Here's how the part is built. I have some questions about the finished solid (model axes, mm). Face numbers are marked on the shaded views. A direction names the side the tool comes from. Coordinates: 2 decimals unless noted, no trailing zeros. Loops run counter-clockwise (first coordinate to the right, second up) from the corner with the lowest first, then second, coordinate; pieces in that order, holes last. Notation, with made-up numbers: (51, -7.5) -> (62, -7.5) arc R7 ccw to (62, 0.5) -> close; hole circle Ø10 at (1.5, -30). An arc over 180 degrees is marked (long way). Answer as a JSON object with one key per item and string values. Group by question number.
Q1. I'm going to push flat-ended pins straight in: pin 1 (2 mm diameter, centred on y = 3, z = 4, fed in from +X); pin 2 (3.5 mm diameter, centred on x = -1, y = -1, fed in from +Z); pin 3 (3 mm diameter, centred on y = -2.5, z = 2.5, fed in from -X); pin 4 (1.8 mm diameter, centred on x = 17, y = 0, fed in from -Z). Where does each tip first touch, or does it pass through?
Q2. I want a section at D-D on z = 2.75. Write out the boundary of the cut face in (x, y), then the cut area to 3 significant figures.
Q3. I want a section at B-B on y = 0. Write out the boundary of the cut face in (x, z).
Q4. On a 3-axis mill with a long thin cutter (end or side, diameter ignored), from which of +Z, -Z, +X, -X, +Y, -Y can I reach the whole of each face in a straight line? I mean the marked faces 4 and 5. Say none if no direction works.
Q5. I want a section at C-C on x = 17. Write out the boundary of the cut face in (y, z).
Q6. Thinking about a two-plate mould opening in X: for the marked faces 1, 2 and 3, which applies, released by +X, released by -X, zero draft, split by the parting line, or undercut?
Q7. I need wall thicknesses on line 1 (Y direction, x = 0, z = 1.4); line 2 (Y direction, x = 0, z = 4.1); line 3 (X direction, y = -1.75, z = 2.65). Which ranges of each line are inside material? Lowest first, please.
Q8. I want a section at A-A on z = 1.05. Write out the boundary of the cut face in (x, y).
```python
from build123d import *

# Parameters (mm, degrees)
SKETCH1_R           = 1.5
BOSS_EXTRUDE1_DEPTH = 2
SKETCH2_R           = 4.5
SKETCH2_R_2         = 3.5
BOSS_EXTRUDE2_DEPTH = 3
SKETCH3_R           = 1
CUT_EXTRUDE1_DEPTH  = 3


with BuildPart() as part:
    # Sketch1 → Boss-Extrude1 (new body)
    with BuildSketch(Plane.XY):
        with BuildLine():
            Line((-17.442345164, 2.460554969), (-3.31662479, 5))
            ThreePointArc((-3.31662479, 5), (0, 6), (3.31662479, 5))
            Line((3.31662479, 5), (17.442345164, 2.460554969))
            ThreePointArc((17.442345164, 2.460554969), (19.5, 0), (17.442345164, -2.460554969))
            Line((17.442345164, -2.460554969), (3.31662479, -5))
            ThreePointArc((3.31662479, -5), (0, -6), (-3.31662479, -5))
            Line((-3.31662479, -5), (-17.442345164, -2.460554969))
            ThreePointArc((-17.442345164, -2.460554969), (-19.5, 0), (-17.442345164, 2.460554969))
        make_face()
        Circle(SKETCH1_R, mode=Mode.SUBTRACT)
    extrude(amount=BOSS_EXTRUDE1_DEPTH)

    # Sketch2 → Boss-Extrude2 (add)
    with BuildSketch(Plane.XY.offset(2)):
        Circle(SKETCH2_R)
        Circle(SKETCH2_R_2, mode=Mode.SUBTRACT)
    extrude(amount=BOSS_EXTRUDE2_DEPTH)

    # Sketch3 → Cut-Extrude1 (cut, through all)
    with BuildSketch(Plane.XY.offset(2)):
        with Locations((-17, 0)):
            Circle(SKETCH3_R)
        with Locations((17, 0)):
            Circle(SKETCH3_R)
    extrude(amount=-CUT_EXTRUDE1_DEPTH, mode=Mode.SUBTRACT)


solid = part.part
```
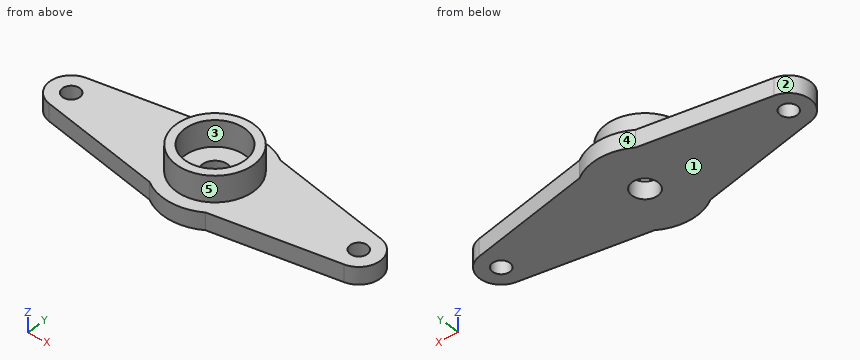
Result set:
{
 "1": {"pin 1": "stops at x = 4.03", "pin 2": "stops at z = 2", "pin 3": "stops at x = -19.25", "pin 4": "passes through"},
 "2": {"outline": "circle Ø9 at (0, 0); hole circle Ø7 at (0, 0)", "area": "25.1 mm²"},
 "3": {"outline": "(-19.5, 0) -> (-18, 0) -> (-18, 2) -> (-19.5, 2) -> close; (-16, 0) -> (-1.5, 0) -> (-1.5, 2) -> (-3.5, 2) -> (-3.5, 5) -> (-4.5, 5) -> (-4.5, 2) -> (-16, 2) -> close; (1.5, 0) -> (16, 0) -> (16, 2) -> (4.5, 2) -> (4.5, 5) -> (3.5, 5) -> (3.5, 2) -> (1.5, 2) -> close; (18, 0) -> (19.5, 0) -> (19.5, 2) -> (18, 2) -> close"},
 "4": {"face 4": "+Z, -Z, +Y", "face 5": "+Z"},
 "5": {"outline": "(-2.54, 0) -> (-1, 0) -> (-1, 2) -> (-2.54, 2) -> close; (1, 0) -> (2.54, 0) -> (2.54, 2) -> (1, 2) -> close"},
 "6": {"face 1": "zero draft", "face 2": "released by -X", "face 3": "undercut"},
 "7": {"line 1": "y = -6 to -1.5, 1.5 to 6", "line 2": "y = -4.5 to -3.5, 3.5 to 4.5", "line 3": "x = -4.15 to -3.03, 3.03 to 4.15"},
 "8": {"outline": "(-17.44, -2.46) -> (-3.32, -5) arc R6 ccw to (3.32, -5) -> (17.44, -2.46) arc R2.5 ccw to (17.44, 2.46) -> (3.32, 5) arc R6 ccw to (-3.32, 5) -> (-17.44, 2.46) arc R2.5 ccw to start; hole circle Ø2 at (-17, 0); hole circle Ø3 at (0, 0); hole circle Ø2 at (17, 0)"}
}
